```python
from build123d import *

# Parameters (mm, degrees)
SKETCH_2_OUTSIDE_W       = 35.526
SKETCH_2_OUTSIDE_H       = 35.526
SKETCH_2_OUTSIDE_W_2     = 12
SKETCH_2_OUTSIDE_H_2     = 28
CUT_EXTRUDE_1_DEPTH      = 9
SKETCH_3_W               = 30
SKETCH_3_H               = 3
CUT_EXTRUDE_2_DEPTH      = 10
CUT_EXTRUDE_2_DEPTH_BACK = 4


with BuildPart() as part:
    # Эскиз1 → Повернуть1 (revolve)
    with BuildSketch(Plane(origin=(0, 0, 0), x_dir=(0, 0, -1), z_dir=(1, 0, 0))):
        with BuildLine():
            Line((13, 1.217734844), (13, 5.246033508))
            ThreePointArc((13, 5.246033508), (6.644251866, 7.303952511), (0, 8))
            Line((0, 8), (0, 0))
            ThreePointArc((0, 0), (6.528454606, 0.305098605), (13, 1.217734844))
        make_face()
    revolve(axis=Axis((0, 8, 0), (0, -1, 0)))

    # Эскиз2 outside → Вырез-Вытянуть1 (cut, through all)
    with BuildSketch(Plane.XZ.offset(-8)):
        Rectangle(SKETCH_2_OUTSIDE_W, SKETCH_2_OUTSIDE_H)
        with Locations((3, 0)):
            Rectangle(SKETCH_2_OUTSIDE_W_2, SKETCH_2_OUTSIDE_H_2, mode=Mode.SUBTRACT)
    extrude(amount=CUT_EXTRUDE_1_DEPTH, mode=Mode.SUBTRACT)

    # Эскиз3 → Вырез-Вытянуть2 (cut, two sides)
    with BuildSketch(Plane(origin=(0, 0, 0), x_dir=(0, 0, -1), z_dir=(1, 0, 0))) as cut_extrude_2_sk:
        with Locations((0, 1.5)):
            Rectangle(SKETCH_3_W, SKETCH_3_H)
    extrude(amount=CUT_EXTRUDE_2_DEPTH, mode=Mode.SUBTRACT)
    extrude(cut_extrude_2_sk.sketch, amount=-CUT_EXTRUDE_2_DEPTH_BACK, mode=Mode.SUBTRACT)


solid = part.part
```
The model under review builds one solid part; all positions refer to its coordinate system, in mm. Coordinates: 2 decimals unless noted, no trailing zeros. Write each loop counter-clockwise with the first axis right and the second up, starting at its lowest first coordinate (ties: lowest second). Pieces come first, ordered by that corner, then holes. Notation, with made-up numbers: (6.25, 49) - (27.25, 49) arc R19 ccw to (27.25, 83) - close; hole circle Ø6 at (-30.75, 77). An arc over 180 degrees is marked (long way). Write item = value, one per line.
(1) Consider section A-A, the plane y = 3.5. Give the boundary of the cut face in (x, z).
Result sheet:
outline = (-3, -12.65) arc R13 ccw to (9, -9.38) - (9, 9.38) arc R13 ccw to (-3, 12.65) - close
(2) For line 1 (Y direction, x = -1.75, z = -2.5); line 2 (Y direction, x = 8, z = 5.75); line 3 (Z direction, x = 4.5, y = 4.65), list the stretches that pass through material, from the lowest coordinate up. Write a range as [from, to].
Result sheet:
line_1 = [3, 7.85]
line_2 = [3, 6.45]
line_3 = [-12.2, 12.2]
(3) Consider section C-C, the plane y = 7.4. Give the boundary of the cut face in (x, z), then the cut area to 3 significant figures.
Result sheet:
outline = (-3, -5.4) arc R6.17 ccw (long way) to (-3, 5.4) - close
area = 95.4 mm^2
(4) Consider section B-B, the plane z = -1. Give the boundary of the cut face in (x, y), then the cut area to 3 significant figures.
Result sheet:
outline = (-3, 3) - (9, 3) - (9, 6.69) arc R32.04 ccw to (-3, 7.84) - close
area = 55.8 mm^2
